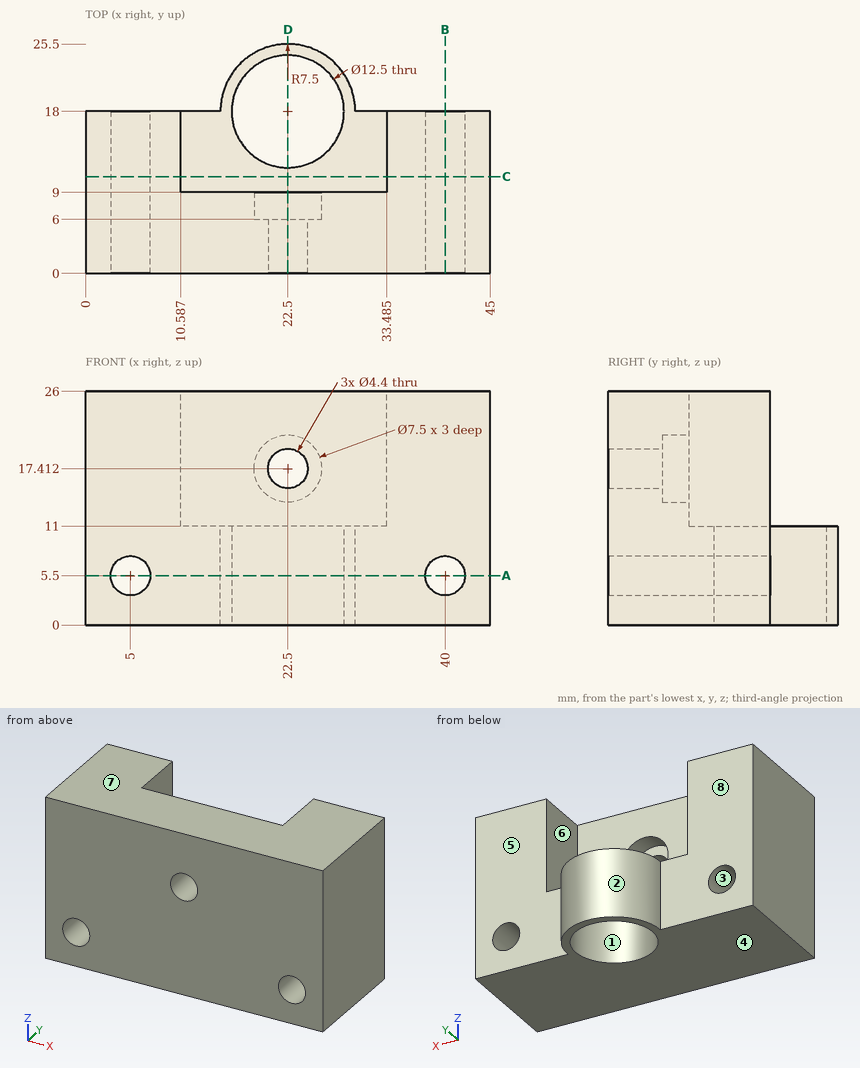
Answer from the drawing. Dimensions are ordinates in mm from the lowest x, y and z of the part. A direction names the side the tool comes from. Round coordinates to 2 decimals unless told otherwise and drop trailing zeros. Loops run counter-clockwise (first coordinate to the right, second up) from the corner with the lowest first, then second, coordinate; pieces in that order, holes last. Notation, with made-up numbers: (52.5, 1.25) - (76.5, 1.25) arc R9 ccw to (76.5, 7.25) - close; hole circle Ø9 at (13, 0). An arc over 180 degrees is marked (long way). One line per item, written item: value.
Q1. Each of these flat-tipped pins is pushed along its axis until it touches: pin 1 Ø12 at (x, z) = (22.5, 17.41) entering from +Y; pin 2 Ø5.5 at (x, z) = (40, 5.5) entering from +Y; pin 3 Ø5 at (x, y) = (20.5, 23) entering from +Z. Where does it stop, or does it pass through?
Check values:
pin 1: y = 9
pin 2: y = 18
pin 3: z = 11
Q2. Straight lines are drawn through the part: probe 1 along Z at (x, y) = (22.5, 6.65); probe 2 along X at (y, z) = (10, 22.5) (1 decimal); probe 3 along Z at (x, y) = (40, 7.75). For each, find the intervals that lie inside material, in ascending order.
Check values:
probe 1: 0 to 13.66, 21.16 to 26
probe 2: 0 to 10.6, 33.5 to 45
probe 3: 0 to 3.3, 7.7 to 26
Q3. Find section A-A on z = 5.5. Give the vertices of the cut face in (x, y), and give its area (3 significant figures).
Check values:
outline: (0, 0) - (2.8, 0) - (2.8, 18) - (0, 18) - close; (7.2, 0) - (37.8, 0) - (37.8, 18) - (30, 18) arc R7.5 ccw to (15, 18) - (7.2, 18) - close; (42.2, 0) - (45, 0) - (45, 18) - (42.2, 18) - close; hole circle Ø12.5 at (22.5, 18)
area: 617 mm2
Q4. The mould has two halves that part along Y. Classify the marked faces 1, 2 and 3: +Y half, -Y half, draft (parallel to the pull), parting line (faces both ways), or undercut.
Check values:
face 1: undercut
face 2: +Y half
face 3: draft
Q5. Find section B-B on x = 40. Give the vertices of the cut face in (y, z).
Check values:
outline: (0, 0) - (18, 0) - (18, 3.3) - (0, 3.3) - close; (0, 7.7) - (18, 7.7) - (18, 26) - (0, 26) - close
Q6. Find section C-C on y = 10.75. Give the vertices of the cut face in (x, z) (1 decimal).
Check values:
outline: (0, 0) - (45, 0) - (45, 26) - (33.5, 26) - (33.5, 11) - (10.6, 11) - (10.6, 26) - (0, 26) - close; hole circle Ø4.4 at (5, 5.5); hole circle Ø4.4 at (40, 5.5)
Q7. Find section D-D on x = 22.5. Give the vertices of the cut face in (y, z).
Check values:
outline: (0, 0) - (11.75, 0) - (11.75, 11) - (9, 11) - (9, 13.66) - (6, 13.66) - (6, 15.21) - (0, 15.21) - close; (0, 19.61) - (6, 19.61) - (6, 21.16) - (9, 21.16) - (9, 26) - (0, 26) - close; (24.25, 0) - (25.5, 0) - (25.5, 11) - (24.25, 11) - close
Q8. For the marked faces 4, 5, 6, 7 and 8, determine the directions among +Z, -Z, +X, -X, +Y, -Y from which every point of the face is accessible in a straight line to the end or side of a thin tool.
Check values:
face 4: -Z, +X, -X, +Y, -Y
face 5: +Z, -Z, +X, +Y
face 6: +Z, +Y
face 7: +Z, +X, -X, +Y, -Y
face 8: +Z, -Z, -X, +Y
